```python
from build123d import *

# Parameters (mm, degrees)
SKETCH2_W           = 120
SKETCH2_H           = 35
SKETCH2_R           = 1.5
SKETCH2_R_2         = 3.965
BOSS_EXTRUDE1_DEPTH = 10


with BuildPart() as part:
    # Sketch2 → Boss-Extrude1 (new body)
    with BuildSketch(Plane.XY):
        with Locations((26.590909091, -2.670454545)):
            Rectangle(SKETCH2_W, SKETCH2_H)
        with Locations((-29.873557003, -16.63492064)):
            Circle(SKETCH2_R, mode=Mode.SUBTRACT)
        with Locations((-15.909090909, -2.670454545)):
            Circle(SKETCH2_R_2, mode=Mode.SUBTRACT)
        with Locations((83.055375185, 11.294011549)):
            Circle(SKETCH2_R, mode=Mode.SUBTRACT)
        with Locations(Location((-29.873557003, 11.294011549, 0), (0, 0, 180))):
            Circle(SKETCH2_R, mode=Mode.SUBTRACT)
        with Locations(Location((83.055375185, -16.63492064, 0), (0, 0, 180))):
            Circle(SKETCH2_R, mode=Mode.SUBTRACT)
    extrude(amount=BOSS_EXTRUDE1_DEPTH)


solid = part.part
```
Could you check a few things on this model? Use its own coordinates, in mm. Round coordinates to 2 decimals unless told otherwise and drop trailing zeros. Loops run counter-clockwise (first coordinate to the right, second up) from the corner with the lowest first, then second, coordinate; pieces in that order, holes last. Notation, with made-up numbers: (6, 28) - (54, 28) arc R25 ccw to (54, 66) - close; hole circle Ø9 at (-5, 57.5). An arc over 180 degrees is marked (long way). Use CSV: the item, a comma, the result in double quotes.
Item 1: If we section it at B-B on z = 2.25: List the corners of the cut face in (x, y) for me (3 decimals), then the cut area to 3 significant figures.
Here are the results:
outline,"(-33.409, -20.17) - (86.591, -20.17) - (86.591, 14.83) - (-33.409, 14.83) - close; hole circle Ø3 at (-29.874, -16.635); hole circle Ø3 at (-29.874, 11.294); hole circle Ø7.93 at (-15.909, -2.67); hole circle Ø3 at (83.055, -16.635); hole circle Ø3 at (83.055, 11.294)"
area,"4,120 mm²"
Item 2: If we section it at A-A on x = -13.5: List the corners of the cut face in (y, z) for me, then the cut area to 3 significant figures.
Here are the results:
outline,"(-20.17, 0) - (-5.82, 0) - (-5.82, 10) - (-20.17, 10) - close; (0.48, 0) - (14.83, 0) - (14.83, 10) - (0.48, 10) - close"
area,"287 mm²"
Item 3: If we mould it in two halves opening along X, with no side actions, what happens to faces 1 (the cylindrical face through (84.554, -16.701, 4.93)), 2 (the flat face through (26, 14.83, 5)), 3 (the cylindrical face through (84.5, 11.7, 4.9)), 4 (the flat face through (86.591, -3, 5))? For each: pulls with the +X half, pulls with the -X half, needs draft (parallel to the pull), parting line crosses it, or undercut.
Here are the results:
face 1,"undercut"
face 2,"needs draft"
face 3,"undercut"
face 4,"pulls with the +X half"
Item 4: Will this pin go through, and if not, where does the flat tip stop? pin 1 (1.8 mm diameter, centred on x = -29.87, y = -16.63, fed in from -Z).
Here are the results:
pin 1,"passes through"
Item 5: I need wall thicknesses on L1, parallel to X at y = -18, z = 2; L2, parallel to X at y = -15.5, z = 9.25; L3, parallel to X at y = -3, z = 3.5. Which ranges of each line are inside material? Lowest first, please. Write a range as [from, to].
Here are the results:
L1,"x = [-33.41, -30.5], [-29.25, 82.43], [83.68, 86.59]"
L2,"x = [-33.41, -30.85], [-28.89, 82.07], [84.04, 86.59]"
L3,"x = [-33.41, -19.86], [-11.96, 86.59]"
